```python
from build123d import *

# Parameters (mm, degrees)
F0_R     = 4.25
F1_DEPTH = 21
F2_DEPTH = 6
F3_R     = 7.5
F3_R_2   = 4.25
F4_DEPTH = 2.5
F6_DEPTH = 18
F7_R     = 0.5
F8_R     = 1


with BuildPart() as f1:
    # F0 (on Front) → F1 (new body)
    with BuildSketch(Plane.XZ):
        Circle(F0_R)
        Polygon((-1.125, 1.948557), (2.25, 0), (-1.125, -1.948557), align=None, mode=Mode.SUBTRACT)
        Polygon((-1.125, -1.948557), (2.25, 0), (-1.125, 1.948557), align=None)
    extrude(amount=F1_DEPTH)

    # F0 (on Front) → F2 (join)
    with BuildSketch(Plane.XZ):
        Polygon((-1.125, -1.948557), (2.25, 0), (-1.125, 1.948557), align=None)
    extrude(amount=-F2_DEPTH)

    # F3 (on face) → F4 (join)
    with BuildSketch(Plane.XZ.offset(21)):
        Circle(F3_R)
        Circle(F3_R_2, mode=Mode.SUBTRACT)
        Circle(F3_R_2)
    extrude(amount=F4_DEPTH)

    # F5 (on face) → F6 (join)
    with BuildSketch(Plane.XZ.offset(23.5)):
        Polygon((0.076423, -4.499351), (3.934764, -2.183492), (3.858341, 2.315859), (-0.076423, 4.499351), (-3.934764, 2.183492), (-3.858341, -2.315859), align=None)
    extrude(amount=F6_DEPTH)

    # F7
    f7_edges = [f1.edges().sort_by_distance(p)[0] for p in [
        (2.005593, -41.5, -3.341421),
        (-1.890959, -41.5, -3.407605),
        (-3.896552, -41.5, -0.066184),
        (-2.005593, -41.5, 3.341421),
        (1.890959, -41.5, 3.407605),
        (3.896552, -41.5, 0.066184),
    ]]
    fillet(f7_edges, radius=F7_R)

    # F8
    f8_edges = [f1.edges().sort_by_distance(p)[0] for p in [
        (-7.5, -23.5, 0),
        (-7.5, -21, 0),
    ]]
    fillet(f8_edges, radius=F8_R)


solid = f1.part
```
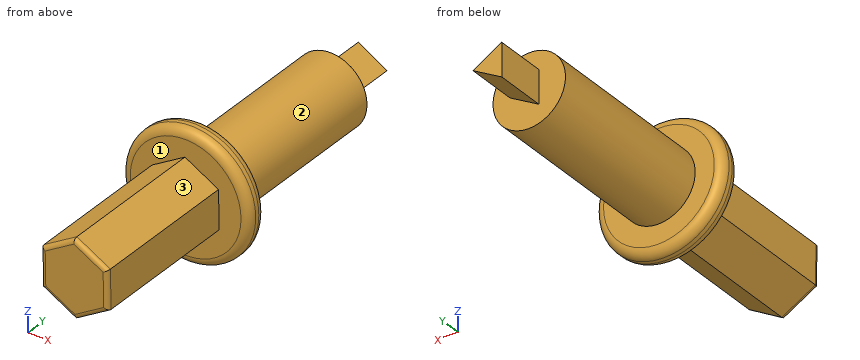
Source: CAD feature listing. Evaluate the final solid. Frame: model axes, mm. Face numbers are marked on the shaded views. A direction names the side the tool comes from. Round coordinates to 2 decimals unless told otherwise and drop trailing zeros. Write each loop counter-clockwise with the first axis right and the second up, starting at its lowest first coordinate (ties: lowest second). Pieces come first, ordered by that corner, then holes. Notation, with made-up numbers: M -0.5,42 L 18.5,42 A33 ccw 18.5,76 Z; hole C -10,13 d10. An arc over 180 degrees is marked long. Answer as a JSON object with one key per item and string values. Group by question number.
(1) Section query A-A on y = -33. Output: boundary loops of the cut face in (x, z), then the cut area to 3 significant figures.
(2) First-contact query: pin 1 (1.5 mm diameter, centred on x = -4.5, y = -19, fed in from -Z); pin 2 (8 mm diameter, centred on x = 2, z = 4, fed in from -Y); pin 3 (5 mm diameter, centred on x = -3.5, y = -8, fed in from +Z); pin 4 (1 mm diameter, centred on y = -35, z = -2.5, fed in from -X). Flat tips, straight axial feed; report the tip coordinate or a pass-through.
(3) Ray query, line 1 (Y direction, x = -0.25, z = 6.25); line 2 (Y direction, x = -2, z = 0.5); line 3 (Z direction, x = 2.5, y = -22). Return the intervals inside material, ascending. Write a range as [from, to].
(4) Reachability of the marked faces 1, 2 and 3 from +Z, -Z, +X, -X, +Y, -Y: full face, straight path, thin tool, end or side. Return the list, or none.
(5) Section query B-B on y = -16. Output: boundary loops of the cut face in (x, z), then the cut area to 3 significant figures.
Computed values:
{
 "1": {"outline": "M -3.93,2.18 L -3.86,-2.32 L 0.08,-4.5 L 3.93,-2.18 L 3.86,2.32 L -0.08,4.5 Z", "area": "52.6 mm^2"},
 "2": {"pin 1": "z = -2", "pin 2": "y = -41.5", "pin 3": "z = 4.13", "pin 4": "x = -3.86"},
 "3": {"line 1": "[-23.5, -21]", "line 2": "[-41.5, 0]", "line 3": "[-7.07, 7.07]"},
 "4": {"face 1": "-Y", "face 2": "+Y", "face 3": "+Z, +X, -Y"},
 "5": {"outline": "C 0,0 d8.5", "area": "56.7 mm^2"}
}
